Geometry check sheet. Reference: the model listing, model coordinates, mm. A direction names the side the tool comes from. Give positions to 0.01 mm unless a question says otherwise; leave off trailing zeros. One line per item, written item: value. Start each with the question number.
(1) Draft check along Z on faces 5 (the face through (28, -8.594, 0)), 6 (the face through (-265.38, 6.1, -217.15)), 7 (the face through (19, 0, 12.7)), 8 (the face through (-122.368, 0.363, 49.076)). Enter one of: pulls with the +Z half, pulls with the -Z half, needs draft (parallel to the pull), parting line crosses it, or undercut.
(2) Scan lines: line 1 along Y through (x, z) = (-157, -120); line 2 along Z through (x, y) = (14.5, 0); line 3 along Z through (x, y) = (-56, -0.5). Record each from-to range of solid material in increasing order. Write a range as from..to.
(3) Gauge pin test, flat ends, axial feed: pin 1 Ø2 at (x, y) = (-55, 4.5) entering from +Z; pin 2 Ø8.5 at (y, z) = (4, -4) entering from +X; pin 3 Ø1.5 at (y, z) = (-6.5, -171) entering from +X. Record the tip position at first contact, or that the pin passes through.
(4) Tool access check on faces 1 (the face through (19, 0, -12.7)), 2 (the face through (21.005, 0, 0)), 3 (the face through (-265.38, -6.14, -217.15)), 4 (the face through (-267, -4.761, -219)). Record the directions out of +Z, -Z, +X, -X, +Y, -Y that give a thin tool (end or side, any length) a straight path to the whole face; none if there is none.
from build123d import *

# Parameters (mm, degrees)
SKETCH2_R                = 8.255
BOSS_EXTRUDE1_DEPTH      = 12.7
BOSS_EXTRUDE1_DEPTH_BACK = 12.7
BOSS_EXTRUDE2_DEPTH      = 12.7
BOSS_EXTRUDE2_DEPTH_BACK = 12.7
SKETCH4_W                = 27.044091096
SKETCH4_H                = 9.871476176
BOSS_EXTRUDE3_DEPTH      = 12.7
BOSS_EXTRUDE3_DEPTH_BACK = 12.7
SKETCH5_W                = 22.839690924
SKETCH5_H                = 9.521004572


with BuildPart() as part:
    # Sweep1: sweep along a path in Sketch1
    with BuildLine(Plane(origin=(0, 0, 0), x_dir=(1, 0, 0), z_dir=(0, 1, 0))) as sweep1_path:
        Line((-265.319834303, -87.577083333), (0, 0))
        Line((0, 0), (-265.319834303, 217.222916667))
    # Sketch2 → Sweep1 (sweep)
    with BuildSketch(Plane(origin=(-265.319834303, 0, 87.577083333), x_dir=(-0.3134469696969697, 0, -0.949605706168506), z_dir=(0.949605706168506, 0, -0.3134469696969697))):
        Circle(SKETCH2_R)
    sweep(path=sweep1_path.line, transition=Transition.RIGHT)

    # Sketch3 → Boss-Extrude1 (add, two sides: drawn at the far end of the back side and taken through both)
    with BuildSketch(Plane.XY.offset(-BOSS_EXTRUDE1_DEPTH_BACK)):
        Polygon((33.931753368, 15.31554454), (13.629365652, 15.31554454), (13.629365652, -15.31554454), (33.931753368, -15.31554454), (33.931753368, -8.593796811), (21.004584429, -8.593796811), (21.004584429, 8.593796811), (33.931753368, 8.593796811), align=None)
    extrude(amount=BOSS_EXTRUDE1_DEPTH + BOSS_EXTRUDE1_DEPTH_BACK)

    # Sketch4 → Boss-Extrude2 (add, two sides: drawn at the far end of the back side and taken through both)
    with BuildSketch(Plane(origin=(-265.319834303, 0, 87.577083333), x_dir=(0.3134469696969697, 0, 0.949605706168506), z_dir=(-0.949605706168506, 0, 0.3134469696969697)).offset(-BOSS_EXTRUDE2_DEPTH_BACK)):
        Rectangle(SKETCH4_W, SKETCH4_H)
    extrude(amount=BOSS_EXTRUDE2_DEPTH + BOSS_EXTRUDE2_DEPTH_BACK)

    # Sketch5 → Boss-Extrude3 (add, two sides: drawn at the far end of the back side and taken through both)
    with BuildSketch(Plane(origin=(-265.319834303, 0, -217.222916667), x_dir=(-0.633487654320988, 0, 0.7737527976187824), z_dir=(-0.7737527976187824, 0, -0.633487654320988)).offset(-BOSS_EXTRUDE3_DEPTH_BACK)):
        Rectangle(SKETCH5_W, SKETCH5_H)
    extrude(amount=BOSS_EXTRUDE3_DEPTH + BOSS_EXTRUDE3_DEPTH_BACK)


solid = part.part
Calculated:
1. face 5: needs draft
1. face 6: pulls with the -Z half
1. face 7: pulls with the +Z half
1. face 8: undercut
2. line 1: y = -4.95..4.95
2. line 2: z = -12.7..12.7
2. line 3: z = -56.5..-35.2, 9.81..27.16
3. pin 1: stops at z = 26.13
3. pin 2: stops at x = 21
3. pin 3: stops at x = -199.2
4. face 1: -Z, +X, +Y, -Y
4. face 2: +Z, -Z, +X
4. face 3: -Z, -X, -Y
4. face 4: -Y
